from build123d import *

# Parameters (mm, degrees)
F0_R          = 1.7
F1_DEPTH      = 1.5
F1_DEPTH_BACK = 6
F2_DEPTH      = 6
F3_T1_DEPTH   = 22
F3_T3_DEPTH   = 40.7


# Not quite as in the source:
# - a fillet or chamfer that OpenCascade refuses, or shapes differently, is made with other operations: its cross-section is extruded or revolved along the edge and cut away or added


with BuildPart() as f1:
    # F0 (on Top) → F1 (new body, two sides)
    with BuildSketch(Plane.XY) as f1_sk:
        Polygon((-4.7234346752, 0.4355579215), (-4.7234346752, -9.1929948391), (-2.7234009317, -14.6884420785), (2.9765315813, -14.6884420785), (4.9765653248, -9.1929948391), (4.9765653248, 0.4355579215), (4.9765653248, 10.028440195), (1.9944189816, 13.0115579215), (0.1265653248, 13.0115579215), (-1.7412883319, 13.0115579215), (-4.7234346752, 10.028440195), align=None)
        with Locations((0.1265653248, 0.4355579215)):
            Circle(F0_R, mode=Mode.SUBTRACT)
    extrude(amount=-F1_DEPTH)
    extrude(f1_sk.sketch, amount=F1_DEPTH_BACK)

    # F0 (on Top) → F2 (join)
    with BuildSketch(Plane.XY):
        Polygon((-8.5234346752, -17.6884420785), (0.1265653248, -17.6884420785), (4.9765653248, -17.6884420785), (8.4765653248, -17.6884420785), (8.4765653248, 18.0115579215), (-8.5234346752, 18.0115579215), align=None)
        Polygon((-2.7234009317, -14.6884420785), (-4.7234346752, -9.1929948391), (-4.7234346752, 0.4355579215), (-4.7234346752, 10.028440195), (-1.7412883319, 13.0115579215), (0.1265653248, 13.0115579215), (1.9944189816, 13.0115579215), (4.9765653248, 10.028440195), (4.9765653248, 0.4355579215), (4.9765653248, -9.1929948391), (2.9765315813, -14.6884420785), align=None, mode=Mode.SUBTRACT)
    extrude(amount=F2_DEPTH)

    # F3: fillet of radius 1 on 4 edges, made by hand

    # F3_s2 → F3_t1 (cut)
    with BuildSketch(Plane.YZ.offset(-11.0234346752)):
        with BuildLine():
            add(Edge.make_bspline(
                [(18.0115579215, 5), (18.0115579215, 6), (17.0115579215, 6)],
                knots=[0, 0, 0, 1, 1, 1], degree=2, weights=[1, 1, 1]))
            Line((17.0115579215, 6), (18.0115579215, 6))
            Line((18.0115579215, 6), (18.0115579215, 5))
        make_face()
        with BuildLine():
            add(Edge.make_bspline(
                [(-17.6884420785, 5), (-17.6884420785, 6), (-16.6884420785, 6)],
                knots=[0, 0, 0, 1, 1, 1], degree=2, weights=[1, 1, 1]))
            Line((-16.6884420785, 6), (-17.6884420785, 6))
            Line((-17.6884420785, 6), (-17.6884420785, 5))
        make_face()
    extrude(amount=F3_T1_DEPTH, mode=Mode.SUBTRACT)

    # F3_s4 → F3_t3 (cut)
    with BuildSketch(Plane.XZ.offset(-20.5115579215)):
        with BuildLine():
            add(Edge.make_bspline(
                [(-8.5234346752, 5), (-8.5234346752, 6), (-7.5234346752, 6)],
                knots=[0, 0, 0, 1, 1, 1], degree=2, weights=[1, 1, 1]))
            Line((-7.5234346752, 6), (-8.5234346752, 6))
            Line((-8.5234346752, 6), (-8.5234346752, 5))
        make_face()
        with BuildLine():
            add(Edge.make_bspline(
                [(8.4765653248, 5), (8.4765653248, 6), (7.4765653248, 6)],
                knots=[0, 0, 0, 1, 1, 1], degree=2, weights=[1, 1, 1]))
            Line((7.4765653248, 6), (8.4765653248, 6))
            Line((8.4765653248, 6), (8.4765653248, 5))
        make_face()
    extrude(amount=F3_T3_DEPTH, mode=Mode.SUBTRACT)


solid = f1.part
The listing builds one solid part. Answer for the finished solid, in the listing's coordinates (mm). A direction names the side the tool comes from. Coordinates: 2 decimals unless noted, no trailing zeros. Loops run counter-clockwise (first coordinate to the right, second up) from the corner with the lowest first, then second, coordinate; pieces in that order, holes last.
1) Determine the mould class of faces 1 (the face through (-3.74, -11.9, -0.76)), 2 (the face through (-2, 0, 6)), 3 (the face through (1.04, 1.87, 2.2)) for opening direction X: pulls with the +X half, pulls with the -X half, needs draft (parallel to the pull), parting line crosses it, or undercut.
2) A tool of negligible diameter and unlimited length cuts with its end or side. For faces 4 (the face through (-6, 0, 0)), 5 (the face through (4.977, 0, -1)), 6 (the face through (-3.21, 11.54, -0.76)), 7 (the face through (3.963, -11.979, -0.76)), 8 (the face through (0, 13.012, -1)), from which of +Z, -Z, +X, -X, +Y, -Y can it reach the whole face along a straight path? Write none if from no direction.
3) Flat-ended cylindrical pins translate along their axes: pin 1 Ø1.2 at (y, z) = (1.5, -1) entering from +X; pin 2 Ø0.8 at (x, z) = (0.5, -1) entering from +Y; pin 3 Ø0.8 at (x, z) = (1.5, -0.5) entering from -Y; pin 4 Ø4 at (x, y) = (0.13, 0.44) entering from -Z. Find the tip coordinate at first contact, or state that the pin passes through.
4) Find the intervals of material crossed by L1, parallel to X at y = 0.5, z = 1; L2, parallel to Z at x = -7.25, y = 13; L3, parallel to Y at x = 1, z = 2, in increasing order.
5) Find section A-A on z = -0.5. Write down the section's boundary in (x, y).
Values:
1. face 1: pulls with the -X half
1. face 2: needs draft
1. face 3: undercut
2. face 4: -Z
2. face 5: -Z, +X, +Y, -Y
2. face 6: -Z, -X, +Y
2. face 7: -Z, +X, -Y
2. face 8: -Z, +X, -X, +Y
3. pin 1: stops at x = 4.98
3. pin 2: stops at y = 13.01
3. pin 3: stops at y = -14.69
3. pin 4: stops at z = -1.5
4. L1: x = -8.52 to -1.57, 1.83 to 8.48
4. L2: z = 0 to 6
4. L3: y = -17.69 to -1.02, 1.89 to 18.01
5. outline: (-4.72, -9.19) - (-2.72, -14.69) - (2.98, -14.69) - (4.98, -9.19) - (4.98, 10.03) - (1.99, 13.01) - (-1.74, 13.01) - (-4.72, 10.03) - close; hole circle Ø3.4 at (0.13, 0.44)
